The listing builds one solid part. Answer for the finished solid, in the listing's coordinates (mm). A direction names the side the tool comes from. Give positions to 0.01 mm unless a question says otherwise; leave off trailing zeros. Write each loop counter-clockwise with the first axis right and the second up, starting at its lowest first coordinate (ties: lowest second). Pieces come first, ordered by that corner, then holes. Notation, with made-up numbers: (78, 22) -> (120, 22) arc R14 ccw to (120, 40) -> close; hole circle Ø5 at (17, 57). An arc over 180 degrees is marked (long way). Put each result on its own line as item: value. Start each with the question number.
1) Flat-ended cylindrical pins translate along their axes: pin 1 Ø10 at (x, z) = (40.5, -16.5) entering from +Y; pin 2 Ø6.5 at (x, z) = (26.55, -14.478) entering from -Y. Find the tip coordinate at first contact, or state that the pin passes through.
2) A cutting plane is placed at D-D (z = -26). Write down the section's boundary in (x, y) (3 decimals), then the cut area to 3 significant figures.
3) Find the intervals of material crossed by line 1 along X through (y, z) = (3.5, -1) (3 decimals); line 2 along Z through (x, y) = (26.55, -2.15); line 3 along Y through (x, z) = (45, -20.5) (3 decimals), in increasing order. Write a range as from..to.
4) A cutting plane is placed at C-C (z = -12.5). Write down the section's boundary in (x, y) (3 decimals), then the cut area to 3 significant figures.
5) For a pull along Z with two mould halves and no side action, classify faces 1 (the flat face through (26, -1, 0)), 2 (the flat face through (53.1, 15, -17)), 3 (the cylindrical face through (23.21, -1.61, -15.53)) as released by +Z, released by -Z, zero draft, split by the parting line, or undercut.
6) For faces 4 (the flat face through (1.565, 25.133, -14.275)), 5 (the cylindrical face through (49.02, 0.955, -14.275)), determine the directions among +Z, -Z, +X, -X, +Y, -Y from which every point of the face is accessible in a straight line to the end or side of a thin tool.
7) A cutting plane is placed at A-A (x = 26.55). Write down the section's boundary in (y, z) (3 decimals), then the cut area to 3 significant figures.
8) A cutting plane is placed at B-B (y = 4). Write down the section's boundary in (x, z) (3 decimals).
from build123d import *

# Parameters (mm, degrees)
SKETCH3_W                      = 53.099999972
SKETCH3_H                      = 28.956
BASE_FLANGE1_DEPTH             = 3.175
EDGE_FLANGE4_STRIP_W           = 19.05
EDGE_FLANGE4_STRIP_H           = 3.175
EDGE_FLANGE4_STRIP_CUT_DEPTH   = 28.956
EDGE_FLANGE4_STRIP_2_W         = 19.05
EDGE_FLANGE4_STRIP_2_H         = 3.175
EDGE_FLANGE4_STRIP_CUT_2_DEPTH = 28.956
EDGE_FLANGE4_DEPTH             = 28.956
EDGE_FLANGE4_FLAT_DEPTH        = 3.175
EDGE_FLANGE4_BEND_DEPTH        = 28.956
EDGE_FLANGE4_FLAT_2_DEPTH      = 3.175
M6_CLEARANCE_HOLE1_D           = 7


# Sheet-metal steps are written as plain solids
with BuildPart() as part:
    # Sketch3 → Base-Flange1 (new body)
    with BuildSketch(Plane(origin=(0, 0, 0), x_dir=(1, 0, 0), z_dir=(0, 1, 0))):
        with Locations((26.549999986, 14.478)):
            Rectangle(SKETCH3_W, SKETCH3_H)
    extrude(amount=-BASE_FLANGE1_DEPTH)

    # Edge-Flange4 strip (across the edge) → Edge-Flange4 strip cut (cut)
    with BuildSketch(Plane(origin=(53.099999972, 0, 0), x_dir=(-1, 0, 0), z_dir=(0, 0, -1))):
        with Locations((-3.175, -1.5875)):
            Rectangle(EDGE_FLANGE4_STRIP_W, EDGE_FLANGE4_STRIP_H)
    extrude(amount=EDGE_FLANGE4_STRIP_CUT_DEPTH, mode=Mode.SUBTRACT)

    # Edge-Flange4 strip 2 (across the edge) → Edge-Flange4 strip cut 2 (cut)
    with BuildSketch(Plane.XY.offset(-28.956)):
        with Locations((-3.175, -1.5875)):
            Rectangle(EDGE_FLANGE4_STRIP_2_W, EDGE_FLANGE4_STRIP_2_H)
    extrude(amount=EDGE_FLANGE4_STRIP_CUT_2_DEPTH, mode=Mode.SUBTRACT)

    # Edge-Flange4 bend section (across the edge) → Edge-Flange4 (add)
    with BuildSketch(Plane(origin=(53.099999972, 0, 0), x_dir=(-1, 0, 0), z_dir=(0, 0, -1))):
        with BuildLine():
            Line((0, 3.175), (3.175, 3.175))
            ThreePointArc((3.175, 3.175), (4.10493597, 0.92993597), (6.35, 0))
            Line((6.35, 0), (6.35, -3.175))
            ThreePointArc((6.35, -3.175), (1.859871939, -1.315128061), (0, 3.175))
        make_face()
    extrude(amount=EDGE_FLANGE4_DEPTH)

    # Edge-Flange4 profile (on flange) → Edge-Flange4 flat (add)
    with BuildSketch(Plane(origin=(53.099999972, 0, 0), x_dir=(0, 0, -1), z_dir=(1, 0, 0))):
        Polygon((0, 6.35), (0, 3.175), (28.956, 3.175), (28.956, 44.45), align=None)
    extrude(amount=-EDGE_FLANGE4_FLAT_DEPTH)

    # Edge-Flange4 bend section 2 (across the edge) → Edge-Flange4 bend (add)
    with BuildSketch(Plane.XY.offset(-28.956)):
        with BuildLine():
            Line((0, 3.175), (3.175, 3.175))
            ThreePointArc((3.175, 3.175), (4.10493597, 0.92993597), (6.35, 0))
            Line((6.35, 0), (6.35, -3.175))
            ThreePointArc((6.35, -3.175), (1.859871939, -1.315128061), (0, 3.175))
        make_face()
    extrude(amount=EDGE_FLANGE4_BEND_DEPTH)

    # Edge-Flange4 profile 2 (on flange) → Edge-Flange4 flat 2 (add)
    with BuildSketch(Plane.ZY):
        Polygon((-28.956, 44.45), (-28.956, 3.175), (0, 3.175), (0, 6.35), align=None)
    extrude(amount=-EDGE_FLANGE4_FLAT_2_DEPTH)

    # M6 Clearance Hole1 (through all)
    with Locations(Plane(origin=(0, 0, 0), x_dir=(1, 0, 0), z_dir=(0, 1, 0))):
        with Locations((26.549999986, 14.478)):
            Hole(M6_CLEARANCE_HOLE1_D / 2)


solid = part.part
Reply:
1. pin 1: stops at y = 0
1. pin 2: passes through
2. outline: (0, 3.175) arc R6.35 ccw to (6.35, -3.175) -> (46.75, -3.175) arc R6.35 ccw to (53.1, 3.175) -> (53.1, 40.561) -> (49.925, 40.561) -> (49.925, 3.175) arc R3.175 cw to (46.75, 0) -> (6.35, 0) arc R3.175 cw to (3.175, 3.175) -> (3.175, 40.561) -> (0, 40.561) -> close
2. area: 413 mm2
3. line 1: x = 0..3.175, 49.925..53.1
3. line 2: z = -28.96..-17.98, -10.98..0
3. line 3: y = -3.175..0
4. outline: (0, 3.175) arc R6.35 ccw to (6.35, -3.175) -> (23.663, -3.175) -> (23.663, 0) -> (6.35, 0) arc R3.175 cw to (3.175, 3.175) -> (3.175, 22.797) -> (0, 22.797) -> close; (29.437, -3.175) -> (46.75, -3.175) arc R6.35 ccw to (53.1, 3.175) -> (53.1, 22.797) -> (49.925, 22.797) -> (49.925, 3.175) arc R3.175 cw to (46.75, 0) -> (29.437, 0) -> close
4. area: 282 mm2
5. face 1: released by +Z
5. face 2: zero draft
5. face 3: undercut
6. face 4: +Z, +X, -X, +Y
6. face 5: +Z, -Z, +Y
7. outline: (-3.175, -28.956) -> (0, -28.956) -> (0, -17.978) -> (-3.175, -17.978) -> close; (-3.175, -10.978) -> (0, -10.978) -> (0, 0) -> (-3.175, 0) -> close
7. area: 69.7 mm2
8. outline: (0, -28.956) -> (3.175, -28.956) -> (3.175, 0) -> (0, 0) -> close; (49.925, -28.956) -> (53.1, -28.956) -> (53.1, 0) -> (49.925, 0) -> close
